Read the model definition and answer for the solid it produces. Units are mm, in the model's axes. Face numbers are marked on the shaded views. A direction names the side the tool comes from. Round coordinates to 2 decimals unless told otherwise and drop trailing zeros. Order: outer loops, then holes, each group sorted by start corner. A loop starts at its lowest first (then second) coordinate and runs counter-clockwise, first axis right, second up. Notation, with made-up numbers: (29.5, 46) - (44.5, 46) arc R14 cw to (44.5, 59) - close; hole circle Ø10 at (39.5, 30). An arc over 180 degrees is marked (long way). Put each result on its own line as item: value. Start each with the question number.
Q1. Find the intervals of material crossed by line 1 along Y through (x, z) = (14, 8.25); line 2 along Y through (x, z) = (3, 6); line 3 along X through (y, z) = (-4.5, 10), in increasing order. Write a range as from..to.
Q2. Section B-B on x = 14 is taken. Give the vertices of the cut face in (y, z), then the cut area to 3 significant figures.
Q3. Section D-D on y = 9 is taken. Give the vertices of the cut face in (x, z), then the cut area to 3 significant figures.
Q4. Which of the six approach directions +Z, -Z, +X, -X, +Y, -Y give full straight-line access (tool end or side, diameter ignored) to the marked faces 4 and 5?
Q5. For a pull along Y with two mould halves and no side action, classify the marked faces 1, 2 and 3 as pulls with the +Y half, pulls with the -Y half, needs draft (parallel to the pull), parting line crosses it, or undercut.
Q6. Section A-A on y = 0 is taken. Give the vertices of the cut face in (x, z), then the cut area to 3 significant figures.
Q7. Section C-C on z = 3.5 is taken. Give the vertices of the cut face in (x, y), then the cut area to 3 significant figures.
from build123d import *

# Parameters (mm, degrees)
IZIM1_W                     = 36
IZIM1_H                     = 28
Y_KSEKLIK_EKSTR_ZYON1_DEPTH = 15
IZIM3_R                     = 6
IZIM3_R_2                   = 1.5
KES_EKSTR_ZYON1_DEPTH       = 16
KES_EKSTR_ZYON2_REACH       = 38
IZIM4_R                     = 3.022097143


with BuildPart() as part:
    # Çizim1 → Yükseklik-Ekstrüzyon1 (new body)
    with BuildSketch(Plane.XY):
        Rectangle(IZIM1_W, IZIM1_H)
    extrude(amount=Y_KSEKLIK_EKSTR_ZYON1_DEPTH)

    # Çizim3 → Kes-Ekstrüzyon1 (cut, through all)
    with BuildSketch(Plane.XY.offset(15)):
        with Locations((3, 0)):
            Circle(IZIM3_R)
        with Locations((-9, 0)):
            Circle(IZIM3_R_2)
        with Locations((14, 9)):
            Circle(IZIM3_R_2)
    extrude(amount=-KES_EKSTR_ZYON1_DEPTH, mode=Mode.SUBTRACT)

    # Çizim4 → Kes-Ekstrüzyon2 (cut, up to next)
    with BuildSketch(Plane(origin=(18, 0, 0), x_dir=(0, 0, -1), z_dir=(1, 0, 0)), mode=Mode.PRIVATE) as kes_ekstr_zyon2_sk1:
        with Locations((-7.5, 0)):
            Circle(IZIM4_R)
    kes_ekstr_zyon2_tool1 = extrude(kes_ekstr_zyon2_sk1.sketch, amount=-KES_EKSTR_ZYON2_REACH, mode=Mode.PRIVATE) & part.part
    add(kes_ekstr_zyon2_tool1.solids().sort_by_distance((18, 0, 7.5))[0], mode=Mode.SUBTRACT)


solid = part.part
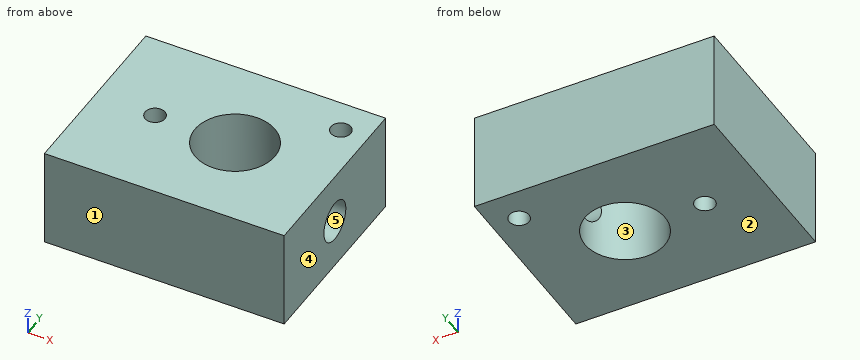
Findings:
1. line 1: -14..-2.93, 2.93..7.5, 10.5..14
1. line 2: -14..-6, 6..14
1. line 3: -18..-0.97, 6.97..18
2. outline: (-14, 0) - (7.5, 0) - (7.5, 15) - (-14, 15) - close; (10.5, 0) - (14, 0) - (14, 15) - (10.5, 15) - close; hole circle Ø6.04 at (0, 7.5)
2. area: 346 mm2
3. outline: (-18, 0) - (12.5, 0) - (12.5, 15) - (-18, 15) - close; (15.5, 0) - (18, 0) - (18, 15) - (15.5, 15) - close
3. area: 495 mm2
4. face 4: +Z, -Z, +X, +Y, -Y
4. face 5: +X
5. face 1: pulls with the -Y half
5. face 2: needs draft
5. face 3: undercut
6. outline: (-18, 0) - (-10.5, 0) - (-10.5, 15) - (-18, 15) - close; (-7.5, 0) - (-3, 0) - (-3, 15) - (-7.5, 15) - close; (9, 0) - (18, 0) - (18, 4.48) - (9, 4.48) - close; (9, 10.52) - (18, 10.52) - (18, 15) - (9, 15) - close
6. area: 261 mm2
7. outline: (-18, -14) - (18, -14) - (18, 14) - (-18, 14) - close; hole circle Ø3 at (-9, 0); hole circle Ø12 at (3, 0); hole circle Ø3 at (14, 9)
7. area: 881 mm2
